Part model, mm, in its own coordinate system. Face numbers are marked on the shaded views. Round coordinates to 2 decimals unless told otherwise and drop trailing zeros. Loops run counter-clockwise (first coordinate to the right, second up) from the corner with the lowest first, then second, coordinate; pieces in that order, holes last. Notation, with made-up numbers: (81.25, 70.5) - (139.25, 70.5) arc R13 cw to (139.25, 81.5) - close; hole circle Ø7 at (46.5, -40). An arc over 180 degrees is marked (long way). Write each question's results on one line, items separated by ' | '. Start each with the question number.
(1) Cut at B-B, the plane x = 0. List the corners of the cut face in (y, z).
(2) Drill centre lines: L1, parallel to X at y = 3.85, z = 0; L2, parallel to Y at x = -9, z = -6.25; L3, parallel to X at y = 7.5, z = 0.25. Where is each one in solid material? Low to high.
(3) Cut at C-C, the plane y = 3.75. List the corners of the cut face in (x, z), then the cut area to 3 significant figures.
(4) Cut at A-A, the plane z = 0. List the corners of the cut face in (x, y).
(5) Mould opens along X. For the marked faces 1, 2 and 3 say: released by +X, released by -X, zero draft, split by the parting line, or undercut.
(6) Cut at D-D, the plane y = 7.75. List the corners of the cut face in (x, z).
(7) Flat gauge pins, fed straight in: P1, Ø2, axis at x = 2.5, y = 3, coming from the -Z side; P2, Ø1.5, axis at x = 1, y = 7.5, coming from the +Z side; P3, Ø4.5, axis at x = -16, z = 0, coming from the +Y side; P4, Ø1.5, axis at x = -10.5, z = 6, coming from the +Y side. Where does each tip first touch, or does it go through?
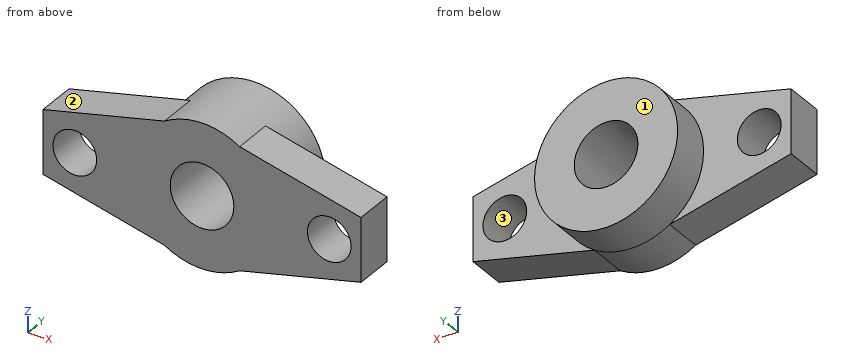
from build123d import *

# Parameters (mm, degrees)
SKETCH1_R           = 9
SKETCH1_R_2         = 4
SKETCH1_R_3         = 2.75
BOSS_EXTRUDE1_DEPTH = 5
SKETCH1_3_R         = 9
SKETCH1_3_R_2       = 4
BOSS_EXTRUDE2_DEPTH = 10


with BuildPart() as part:
    # Sketch1 → Boss-Extrude1 (new body)
    # profile 1 of 3: a face of its own
    with BuildSketch(Plane(origin=(0, 0, 0), x_dir=(1, 0, 0), z_dir=(0, 1, 0))):
        Circle(SKETCH1_R)
        with Locations(Location((0, 0, 0), (0, 0, 270))):
            Circle(SKETCH1_R_2, mode=Mode.SUBTRACT)
    # profile 2 of 3: a face of its own
    with BuildSketch(Plane(origin=(0, 0, 0), x_dir=(1, 0, 0), z_dir=(0, 1, 0))):
        with BuildLine():
            Line((-4.733723721, 7.654531974), (-20, 4))
            Line((-20, 4), (-20, -4))
            Line((-20, -4), (-4.733723721, -7.654531974))
            ThreePointArc((-4.733723721, -7.654531974), (-9, 0), (-4.733723721, 7.654531974))
        make_face()
        with Locations(Location((-16, 0, 0), (0, 0, 270))):
            Circle(SKETCH1_R_3, mode=Mode.SUBTRACT)
    # profile 3 of 3: a face of its own
    with BuildSketch(Plane(origin=(0, 0, 0), x_dir=(1, 0, 0), z_dir=(0, 1, 0))):
        with BuildLine():
            Line((20, 4), (4.733723721, 7.654531974))
            ThreePointArc((4.733723721, 7.654531974), (7.861409336, 4.381579996), (9, 0))
            ThreePointArc((9, 0), (7.861409336, -4.381579996), (4.733723721, -7.654531974))
            Line((4.733723721, -7.654531974), (20, -4))
            Line((20, -4), (20, 4))
        make_face()
        with Locations(Location((16, 0, 0), (0, 0, 270))):
            Circle(SKETCH1_R_3, mode=Mode.SUBTRACT)
    extrude(amount=BOSS_EXTRUDE1_DEPTH)

    # Sketch1_3 → Boss-Extrude2 (add)
    with BuildSketch(Plane(origin=(0, 0, 0), x_dir=(1, 0, 0), z_dir=(0, 1, 0))):
        with Locations(Location((0, 0, 0), (0, 0, 121.733519153))):
            Circle(SKETCH1_3_R)
        with Locations(Location((0, 0, 0), (0, 0, 270))):
            Circle(SKETCH1_3_R_2, mode=Mode.SUBTRACT)
    extrude(amount=BOSS_EXTRUDE2_DEPTH)


solid = part.part
A:
1) outline: (0, -9) - (10, -9) - (10, -4) - (0, -4) - close; (0, 4) - (10, 4) - (10, 9) - (0, 9) - close
2) L1: -20 to -18.75, -13.25 to -4, 4 to 13.25, 18.75 to 20 | L2: 0 to 5 | L3: -9 to -3.99, 3.99 to 9
3) outline: (-20, -4) - (-4.73, -7.65) arc R9 ccw to (4.73, -7.65) - (20, -4) - (20, 4) - (4.73, 7.65) arc R9 ccw to (-4.73, 7.65) - (-20, 4) - close; hole circle Ø5.5 at (-16, 0); hole circle Ø8 at (0, 0); hole circle Ø5.5 at (16, 0) | area: 420 mm2
4) outline: (-20, 0) - (-18.75, 0) - (-18.75, 5) - (-20, 5) - close; (-13.25, 0) - (-4, 0) - (-4, 10) - (-9, 10) - (-9, 5) - (-13.25, 5) - close; (4, 0) - (13.25, 0) - (13.25, 5) - (9, 5) - (9, 10) - (4, 10) - close; (18.75, 0) - (20, 0) - (20, 5) - (18.75, 5) - close
5) face 1: zero draft | face 2: released by -X | face 3: undercut
6) outline: circle Ø18 at (0, 0); hole circle Ø8 at (0, 0)
7) P1: z = -8.87 | P2: z = 9 | P3: through | P4: y = 5
